```python
from build123d import *

# Parameters (mm, degrees)
SKETCH178_R     = 2.6
PAD045_DEPTH    = 4
SKETCH180_R     = 2.6
PAD046_DEPTH    = 5
SKETCH179_R     = 2.6
POCKET098_DEPTH = 5
SKETCH194_R     = 8.1
POCKET109_DEPTH = 8
CHAMFER075_SIZE = 3
CHAMFER076_SIZE = 2
CHAMFER077_SIZE = 1


with BuildPart() as part:
    # Sketch178 → Pad045 (new body)
    with BuildSketch(Plane.XY):
        with BuildLine():
            Line((-32.5531808711, 18.27), (32.5531808711, 18.27))
            ThreePointArc((32.5531808711, 18.27), (33.8522189768, 19.02), (33.8522189768, 20.52))
            Line((26.9240157465, 32.52), (33.8522189768, 20.52))
            ThreePointArc((26.9240157465, 32.52), (24.1788252181, 35.2651905284), (20.4288252181, 36.27))
            Line((-20.4288252181, 36.27), (20.4288252181, 36.27))
            ThreePointArc((-20.4288252181, 36.27), (-24.1788252181, 35.2651905284), (-26.9240157465, 32.52))
            Line((-26.9240157465, 32.52), (-33.8522189768, 20.52))
            ThreePointArc((-33.8522189768, 20.52), (-33.8522189768, 19.02), (-32.5531808711, 18.27))
        make_face()
        with Locations((0, 27.27)):
            Circle(SKETCH178_R, mode=Mode.SUBTRACT)
    extrude(amount=PAD045_DEPTH)

    # Sketch180 → Pad046 (join)
    with BuildSketch(Plane.XY.offset(-5)):
        with BuildLine():
            Line((-32.5531808711, 12.77), (32.5531808711, 12.77))
            ThreePointArc((32.5531808711, 12.77), (38.6153586976, 16.27), (38.6153586976, 23.27))
            Line((31.6871554673, 35.27), (38.6153586976, 23.27))
            ThreePointArc((31.6871554673, 35.27), (26.9288252181, 40.0283302492), (20.4288252181, 41.77))
            Line((-20.4288252181, 41.77), (20.4288252181, 41.77))
            ThreePointArc((-20.4288252181, 41.77), (-26.9288252181, 40.0283302492), (-31.6871554673, 35.27))
            Line((-31.6871554673, 35.27), (-38.6153586976, 23.27))
            ThreePointArc((-38.6153586976, 23.27), (-38.6153586976, 16.27), (-32.5531808711, 12.77))
        make_face()
        with Locations((0, 27.27)):
            Circle(SKETCH180_R, mode=Mode.SUBTRACT)
    extrude(amount=PAD046_DEPTH)

    # Sketch179 → Pocket098 (cut)
    with BuildSketch(Plane.XY.offset(-5)):
        with BuildLine():
            Line((-29.0890792559, 19.77), (29.0890792559, 19.77))
            ThreePointArc((29.0890792559, 19.77), (30.8211300635, 20.77), (30.8211300635, 22.77))
            Line((25.6249776408, 31.77), (30.8211300635, 22.77))
            ThreePointArc((25.6249776408, 31.77), (23.4288252181, 33.9661524227), (20.4288252181, 34.77))
            Line((-20.4288252181, 34.77), (20.4288252181, 34.77))
            ThreePointArc((-20.4288252181, 34.77), (-23.4288252181, 33.9661524227), (-25.6249776408, 31.77))
            Line((-25.6249776408, 31.77), (-30.8211300635, 22.77))
            ThreePointArc((-30.8211300635, 22.77), (-30.8211300635, 20.77), (-29.0890792559, 19.77))
        make_face()
        with Locations((0, 27.27)):
            Circle(SKETCH179_R, mode=Mode.SUBTRACT)
    extrude(amount=POCKET098_DEPTH, mode=Mode.SUBTRACT)

    # Sketch194 → Pocket109 (cut)
    with BuildSketch(Plane.XY):
        with Locations((0, 27.27)):
            Circle(SKETCH194_R)
    extrude(amount=-POCKET109_DEPTH, mode=Mode.SUBTRACT)

    # Chamfer075
    chamfer075_edges = [part.edges().sort_by_distance(p)[0] for p in [
        (0, 35.37, -5),
        (-11.744118, 34.77, -5),
        (11.744118, 34.77, -5),
        (-23.428825, 33.966152, -5),
        (-28.223054, 27.27, -5),
        (-30.82113, 20.77, -5),
        (-16.074245, 19.77, -5),
        (0, 19.17, -5),
        (16.074245, 19.77, -5),
        (30.82113, 20.77, -5),
        (28.223054, 27.27, -5),
        (23.428825, 33.966152, -5),
    ]]
    chamfer(chamfer075_edges, length=CHAMFER075_SIZE)

    # Chamfer076
    chamfer076_edges = [part.edges().sort_by_distance(p)[0] for p in [
        (0, 41.77, -5),
    ]]
    chamfer(chamfer076_edges, length=CHAMFER076_SIZE)

    # Chamfer077
    chamfer077_edges = [part.edges().sort_by_distance(p)[0] for p in [
        (0, 36.27, 4),
    ]]
    chamfer(chamfer077_edges, length=CHAMFER077_SIZE)


solid = part.part
```
Read the model definition and answer for the solid it produces. Units are mm, in the model's axes. A direction names the side the tool comes from. Give positions to 0.01 mm unless a question says otherwise; leave off trailing zeros. Loops run counter-clockwise (first coordinate to the right, second up) from the corner with the lowest first, then second, coordinate; pieces in that order, holes last.
Item 1: The part is cut by section D-D (x = -18). Write down the section's boundary in (y, z).
Item 2: The part is cut by section A-A (x = 0). Write down the section's boundary in (y, z).
Item 3: Find the intervals of material crossed by line 1 along Y through (x, z) = (0, 2.05); line 2 along Z through (x, y) = (-14, 24.5); line 3 along Y through (x, z) = (0, -2), in increasing order.
Item 4: For faces 1 (the flat face through (0.46, 13.76, -3.99)), 2 (the cylindrical face through (-33.863, 19.039, 1.479)), 3 (the conical face through (37.42, 17.06, -4.43)), 4 (the flat face through (16.26, 18.29, -3.48)), 5 (the cylindrical face through (33.84, 19, 1.48)), determine the directions among +Z, -Z, +X, -X, +Y, -Y from which every point of the face is accessible in a straight line to the end or side of a thin tool.
Item 5: Each of these flat-tipped pins is pushed along its axis until it touches: pin 1 Ø1 at (y, z) = (24, -3.5) entering from -X; pin 2 Ø3 at (y, z) = (17, 1) entering from -X; pin 3 Ø1.5 at (x, z) = (3, 1.5) entering from +Y. Where does it stop, or does it pass through?
Item 6: The part is cut by section B-B (z = 1.5). Write down the section's boundary in (x, y), and give its area (3 significant figures).
Item 7: The part is cut by section C-C (y = 26). Write down the section's boundary in (x, z), and give its area (3 significant figures).
Item 8: The mould has two halves that part along X. Classify faces 6 (the flat face through (0, 41.77, -2)), 7 (the cylindrical face through (0.04, 35.37, -0.99)), 8 (the flat face through (12, 34.77, -1)), 9 (the flat face through (29.9, 26.35, 3.51)): released by +X, released by -X, zero draft, split by the parting line, or undercut.
Taken from the geometry:
1. outline: (12.77, -3) - (14.77, -5) - (16.77, -5) - (19.77, -2) - (19.77, 0) - (34.77, 0) - (34.77, -2) - (37.77, -5) - (39.77, -5) - (41.77, -3) - (41.77, 0) - (36.27, 0) - (36.27, 3) - (35.27, 4) - (19.27, 4) - (18.27, 3) - (18.27, 0) - (12.77, 0) - close
2. outline: (12.77, -3) - (14.77, -5) - (16.17, -5) - (19.17, -2) - (19.17, 0) - (24.67, 0) - (24.67, 4) - (19.27, 4) - (18.27, 3) - (18.27, 0) - (12.77, 0) - close; (29.87, 0) - (35.37, 0) - (35.37, -2) - (38.37, -5) - (39.77, -5) - (41.77, -3) - (41.77, 0) - (36.27, 0) - (36.27, 3) - (35.27, 4) - (29.87, 4) - close
3. line 1: y = 18.27 to 24.67, 29.87 to 36.27
3. line 2: z = 0 to 4
3. line 3: y = 12.77 to 19.17, 35.37 to 41.77
4. face 1: -Z, +X, -X, -Y
4. face 2: +Z, -X
4. face 3: -Z, +X
4. face 4: -Z
4. face 5: +Z, +X
5. pin 1: stops at x = -38.26
5. pin 2: stops at x = -39.36
5. pin 3: stops at y = 36.27
6. outline: (-33.85, 20.52) arc R1.5 ccw to (-32.55, 18.27) - (32.55, 18.27) arc R1.5 ccw to (33.85, 20.52) - (26.92, 32.52) arc R7.5 ccw to (20.43, 36.27) - (-20.43, 36.27) arc R7.5 ccw to (-26.92, 32.52) - close; hole circle Ø5.2 at (0, 27.27)
6. area: 1,050 mm2
7. outline: (-37.04, -3) - (-34.73, -5) - (-32.42, -5) - (-28.96, -2) - (-28.96, 0) - (-2.27, 0) - (-2.27, 4) - (-29.53, 4) - (-30.69, 3) - (-30.69, 0) - (-37.04, 0) - close; (2.27, 0) - (28.96, 0) - (28.96, -2) - (32.42, -5) - (34.73, -5) - (37.04, -3) - (37.04, 0) - (30.69, 0) - (30.69, 3) - (29.53, 4) - (2.27, 4) - close
7. area: 292 mm2
8. face 6: zero draft
8. face 7: undercut
8. face 8: undercut
8. face 9: released by +X
